Autodesk Inventor part; units mm, degrees
ref_plane "Plano inicial" through (0, 0, 30) normal (0, 0, 1) x (1, 0, 0)
ref_plane "Plano final" through (0, 0, 120) normal (0, 0, 1) x (1, 0, 0)
ref_plane "Plano de trabalho4" through (0, -15, 30) normal (0, 0, -1) x (-1, 0, 0)
ref_plane "Plano inicial" through (0, 0, 30) normal (0, 0, 1) x (1, 0, 0)
ref_plane "Plano final" through (0, 0, 120) normal (0, 0, 1) x (1, 0, 0)
sketch "Esboço" plane through (0, 0, 0) normal (0, 0, 1) x (1, 0, 0)
  line L0 (-15, -11) -> (-15, 11)
  line L1 (-11, 15) -> (11, 15)
  line L2 (15, 11) -> (15, -11)
  line L3 (11, -15) -> (-11, -15)
  arc A0 (-15, -11) -> (-11, -15) centre (-11, -11) ccw
  arc A1 (15, 11) -> (11, 15) centre (11, 11) ccw
  arc A2 (-11, 15) -> (-15, 11) centre (-11, 11) ccw
  arc A3 (11, -15) -> (15, -11) centre (11, -11) ccw
  arc A4 (-11, 13) -> (-13, 11) centre (-11, 11) ccw
  line L4 (-11, 13) -> (11, 13)
  arc A5 (13, 11) -> (11, 13) centre (11, 11) ccw
  line L5 (13, 11) -> (13, -11)
  arc A6 (11, -13) -> (13, -11) centre (11, -11) ccw
  line L6 (11, -13) -> (-11, -13)
  arc A7 (-13, -11) -> (-11, -13) centre (-11, -11) ccw
  line L7 (-13, -11) -> (-13, 11)
  line L8 (0, 22.1598) -> (0, -22.1598) construction
  line L9 (-22.1598, 0) -> (22.1598, 0) construction
  dimension "d7" = 4
  dimension "d9" = 30
  dimension "d11" = 30
  dimension "d12" = 2
  dimension "d15" = 15
  dimension "d16" = 15
extrude "Corpo" add sketch "Esboço" along normal up to surface (90 mm away) from surface at 30
sketch "Sketch3" plane through (0, 0, 0) normal (0, 0, 1) x (1, 0, 0)
  line L0 (0, 0) -> (10, 0)
ref_plane "Work Plane3" through (0, 0, 0) normal (0, -1, 0) x (1, 0, 0)
sketch "Sketch4" plane through (0, 0, 0) normal (0, -1, 0) x (1, 0, 0)
  line L0 (-2, 30) -> (12, 30)
  line L1 (-2, 120) -> (12, 120)
  dimension "d18" = 90
ref_plane "Plano de trabalho4" through (0, -15, 30) normal (0, 0, -1) x (-1, 0, 0)
split "Dividir1" plane through (0, -15, 30) removes the side toward (0, 0, -1)
ref_plane "Plano de trabalho5" through (0, 435, 120) normal (0, 0, 1) x (1, 0, 0)
split "Dividir2" plane through (0, 435, 120) removes the side toward (0, 0, 1)
equation "\"d7\" = G_IR"
equation "\"d9\" = G_W"
equation "\"d11\" = G_H"
equation "\"d12\" = G_T"
equation "\"d15\" = 0.5 * d9"
equation "\"d16\" = 0.5 * d11"
equation "\"d3\" = G_L"
equation "\"G_W\" = 30"
equation "\"G_H\" = 30"
equation "\"G_T\" = 2"
equation "\"G_IR\" = 4"
equation "\"G_L\" = d18"
properties part number "ISO 10799-2 - 30x30x2 - 90" material "Aço, suave"
Geometry: final body of the model. Coordinates: model frame, mm. A direction names the side the tool comes from. Give positions to 0.01 mm unless a question says otherwise; leave off trailing zeros. Loops run counter-clockwise (first coordinate to the right, second up) from the corner with the lowest first, then second, coordinate; pieces in that order, holes last. Notation, with made-up numbers: (-30, 41) -> (23, 41) arc R12 ccw to (23, 55) -> close; hole circle Ø5 at (20, 16). An arc over 180 degrees is marked (long way). Use one line per item in the form item = value.
Item 1: Section query A-A on y = -5.5. Output: boundary loops of the cut face in (x, z).
A:
outline = (-15, 30) -> (-13, 30) -> (-13, 120) -> (-15, 120) -> close; (13, 30) -> (15, 30) -> (15, 120) -> (13, 120) -> close
Item 2: Access query for faces 4 (the face through (0, -15, 74)), 5 (the face through (12.4, 12.43, 74.37)). Directions: +Z, -Z, +X, -X, +Y, -Y. A direction counts if a zero-diameter tool reaches every point of the face in a straight line with its end or side. Return the directions, or none.
A:
face_4 = +Z, -Z, +X, -X, -Y
face_5 = +Z, -Z
Item 3: Draft query along X for faces 1 (the face through (12.43, -12.4, 74.37)), 2 (the face through (0, 15, 74)), 3 (the face through (-13.859, 13.797, 74.37)). Return one class per face: pulls with the +X half, pulls with the -X half, needs draft (parallel to the pull), parting line crosses it, or undercut.
A:
face_1 = undercut
face_2 = needs draft
face_3 = pulls with the -X half
Item 4: Section query C-C on z = 62. Output: boundary loops of the cut face in (x, y).
A:
outline = (-15, -11) arc R4 ccw to (-11, -15) -> (11, -15) arc R4 ccw to (15, -11) -> (15, 11) arc R4 ccw to (11, 15) -> (-11, 15) arc R4 ccw to (-15, 11) -> close; hole (-13, -11) arc R2 ccw to (-11, -13) -> (11, -13) arc R2 ccw to (13, -11) -> (13, 11) arc R2 ccw to (11, 13) -> (-11, 13) arc R2 ccw to (-13, 11) -> close
Item 5: Line query: probe 1 along Y at (x, z) = (-8, 99); probe 2 along X at (y, z) = (-12.75, 80). Output: solid intervals per line, ascending.
A:
probe_1 = -15 to -13, 13 to 15
probe_2 = -14.6 to -11.97, 11.97 to 14.6
